The model under review builds one solid part; all positions refer to its coordinate system, in mm. Face numbers are marked on the shaded views. A direction names the side the tool comes from. Coordinates: 2 decimals unless noted, no trailing zeros. Loops run counter-clockwise (first coordinate to the right, second up) from the corner with the lowest first, then second, coordinate; pieces in that order, holes last. Notation, with made-up numbers: M 77.5,4.5 L 108.5,4.5 A32 ccw 108.5,38.5 Z; hole C 76,88.25 d5. An arc over 180 degrees is marked long. One line per item, written item: value.
```python
from build123d import *

# Parameters (mm, degrees)
SKETCH1_R           = 2.8
BOSS_EXTRUDE1_DEPTH = 18.5
CUT_EXTRUDE1_DEPTH  = 8
SKETCH3_R           = 1
CUT_EXTRUDE2_DEPTH  = 6
SKETCH5_R           = 7
BOSS_EXTRUDE2_DEPTH = 5


with BuildPart() as part:
    # Sketch1 → Boss-Extrude1 (new, symmetric)
    with BuildSketch(Plane(origin=(0, 0, 0), x_dir=(0, 0, -1), z_dir=(1, 0, 0))):
        Circle(SKETCH1_R)
    extrude(amount=BOSS_EXTRUDE1_DEPTH, both=True)

    # Sketch2 → Cut-Extrude1 (cut)
    with BuildSketch(Plane(origin=(18.5, 0, 0), x_dir=(0, 0, -1), z_dir=(1, 0, 0))):
        with BuildLine():
            Line((-1.85, 2.101784956), (-1.85, -2.101784956))
            ThreePointArc((-1.85, -2.101784956), (-2.8, 0), (-1.85, 2.101784956))
        make_face()
        with BuildLine():
            Line((1.85, 2.101784956), (1.85, -2.101784956))
            ThreePointArc((1.85, -2.101784956), (2.8, 0), (1.85, 2.101784956))
        make_face()
    extrude(amount=-CUT_EXTRUDE1_DEPTH, mode=Mode.SUBTRACT)

    # Sketch3 → Cut-Extrude2 (cut)
    with BuildSketch(Plane(origin=(18.5, 0, 0), x_dir=(0, 0, -1), z_dir=(1, 0, 0))):
        Circle(SKETCH3_R)
    extrude(amount=-CUT_EXTRUDE2_DEPTH, mode=Mode.SUBTRACT)

    # Sketch5 → Boss-Extrude2 (add)
    with BuildSketch(Plane.ZY.offset(18.5)):
        Circle(SKETCH5_R)
    extrude(amount=BOSS_EXTRUDE2_DEPTH)


solid = part.part
```
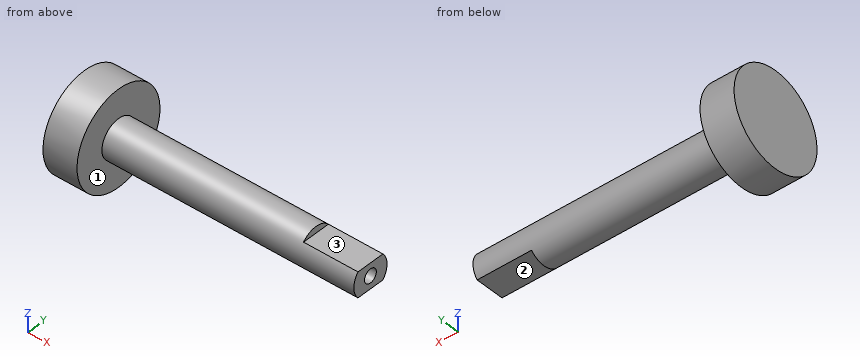
(1) Tool access review of the marked faces 1, 2 and 3: name each direction out of +Z, -Z, +X, -X, +Y, -Y from which nothing blocks a thin tool from reaching the whole face with its end or side.
Checks:
face 1: +X
face 2: -Z, +X, +Y, -Y
face 3: +Z, +X, +Y, -Y
(2) To check wall thickness, follow L1, parallel to Y at x = 14.1, z = 0; L2, parallel to X at y = -5.25, z = 1.75; L3, parallel to Y at x = 2, z = 0. State the ranges of each line that lie inside material, in increasing order. Write a range as [from, to].
Checks:
L1: [-2.8, -1], [1, 2.8]
L2: [-23.5, -18.5]
L3: [-2.8, 2.8]
(3) Add section A-A on z = 0. State the section outline as (x, y) points.
Checks:
outline: M -23.5,-7 L -18.5,-7 L -18.5,-2.8 L 18.5,-2.8 L 18.5,-1 L 12.5,-1 L 12.5,1 L 18.5,1 L 18.5,2.8 L -18.5,2.8 L -18.5,7 L -23.5,7 Z
(4) Insertion check: pin 1 Ø6 at (x, y) = (10.5, 1.5) entering from +Z; pin 2 Ø0.5 at (y, z) = (-1, 2.5) entering from +X; pin 3 Ø4 at (x, y) = (-5.5, 3) entering from +Z; pin 4 Ø0.8 at (y, z) = (-0.5, -2) entering from +X. Each pin has a flat end and moves straight along its axis. Give the tip position at first contact, or say it passes through.
Checks:
pin 1: z = 2.8
pin 2: x = 10.5
pin 3: z = 2.62
pin 4: x = 18.5
(5) Add section C-C on x = 7. State the section outline as (y, z) points.
Checks:
outline: C 0,0 d5.6
(6) Add section B-B on y = 0. State the section outline as (x, z) points, then the cut area to 3 significant figures.
Checks:
outline: M -23.5,-7 L -18.5,-7 L -18.5,-2.8 L 10.5,-2.8 L 10.5,-1.85 L 18.5,-1.85 L 18.5,-1 L 12.5,-1 L 12.5,1 L 18.5,1 L 18.5,1.85 L 10.5,1.85 L 10.5,2.8 L -18.5,2.8 L -18.5,7 L -23.5,7 Z
area: 250 mm^2
(7) Add section D-D on x = 11.5. State the section outline as (y, z) points.
Checks:
outline: M -2.1,-1.85 L 2.1,-1.85 A2.8 ccw 2.1,1.85 L -2.1,1.85 A2.8 ccw Z
